Could you check a few things on this model? Use its own coordinates, in mm. Face numbers are marked on the shaded views. Give positions to 0.01 mm unless a question says otherwise; leave off trailing zeros. Order: outer loops, then holes, each group sorted by start corner. A loop starts at its lowest first (then second) coordinate and runs counter-clockwise, first axis right, second up. Notation, with made-up numbers: (37, 1.25) -> (48, 1.25) arc R15 ccw to (48, 13.25) -> close; hole circle Ø6 at (-34.75, -1). An arc over 180 degrees is marked (long way). Use one line per item in the form item = value. Start each with the question number.
from build123d import *

# Parameters (mm, degrees)
BOSS_EXTRUDE1_DEPTH     = 3.175
SKETCH2_W               = 6.35
SKETCH2_H               = 25.4
BOSS_EXTRUDE2_DEPTH     = 50.8
SKETCH3_R               = 5.207
CUT_EXTRUDE1_DEPTH      = 34.655
CUT_EXTRUDE1_DEPTH_BACK = 297.545
SKETCH4_W               = 50.8
SKETCH4_H               = 19.05
CUT_EXTRUDE2_DEPTH      = 54.975


with BuildPart() as part:
    # Sketch1 → Boss-Extrude1 (new body, symmetric)
    with BuildSketch(Plane(origin=(0, 0, 0), x_dir=(1, 0, 0), z_dir=(0, 1, 0))):
        Polygon((-136.779, 63.5), (-111.379, 63.5), (-12.7, 63.5), (-12.7, 31.75), (12.7, 31.75), (12.7, 63.5), (111.125, 63.5), (111.125, 31.75), (136.525, 31.75), (136.525, 63.5), (161.925, 63.5), (161.925, 34.874677354), (165.1, 34.874677354), (165.1, 14.046677354), (161.925, 14.046677354), (161.925, 10.414), (141.605, 10.414), (141.605, -10.414), (161.925, -10.414), (161.925, -14.046677354), (165.1, -14.046677354), (165.1, -34.874677354), (161.925, -34.874677354), (161.925, -63.5), (121.92, -63.5), (121.92, -57.15), (106.68, -57.15), (106.68, -63.5), (12.7, -63.5), (12.7, -31.75), (-12.7, -31.75), (-12.7, -63.5), (-106.68, -63.5), (-110.5408, -63.5), (-135.9408, -63.5), (-161.925, -63.5), (-161.925, -34.874677354), (-165.1, -34.874677354), (-165.1, -14.046677354), (-161.925, -14.046677354), (-161.925, -10.414), (-141.605, -10.414), (-141.605, 10.414), (-161.925, 10.414), (-161.925, 14.046677354), (-165.1, 14.046677354), (-165.1, 34.874677354), (-161.925, 34.874677354), (-161.925, 63.5), align=None)
    extrude(amount=BOSS_EXTRUDE1_DEPTH, both=True)

    # Sketch2 → Boss-Extrude2 (add, symmetric)
    with BuildSketch(Plane(origin=(0, 0, 0), x_dir=(1, 0, 0), z_dir=(0, 1, 0))):
        with Locations((128.27, 0)):
            Rectangle(SKETCH2_W, SKETCH2_H)
        with Locations((-128.27, 0)):
            Rectangle(SKETCH2_W, SKETCH2_H)
    extrude(amount=BOSS_EXTRUDE2_DEPTH, both=True)

    # Sketch3 → Cut-Extrude1 (cut, two sides)
    with BuildSketch(Plane.ZY.offset(131.445)) as cut_extrude1_sk:
        with Locations((0, 43.18)):
            Circle(SKETCH3_R)
        with Locations((0, -43.18)):
            Circle(SKETCH3_R)
    extrude(amount=CUT_EXTRUDE1_DEPTH, mode=Mode.SUBTRACT)
    extrude(cut_extrude1_sk.sketch, amount=-CUT_EXTRUDE1_DEPTH_BACK, mode=Mode.SUBTRACT)

    # Sketch4 → Cut-Extrude2 (cut, through all)
    with BuildSketch(Plane(origin=(0, 3.175, 0), x_dir=(1, 0, 0), z_dir=(0, 1, 0))):
        with Locations((-50.8, 53.975)):
            Rectangle(SKETCH4_W, SKETCH4_H)
    extrude(amount=-CUT_EXTRUDE2_DEPTH, mode=Mode.SUBTRACT)


solid = part.part
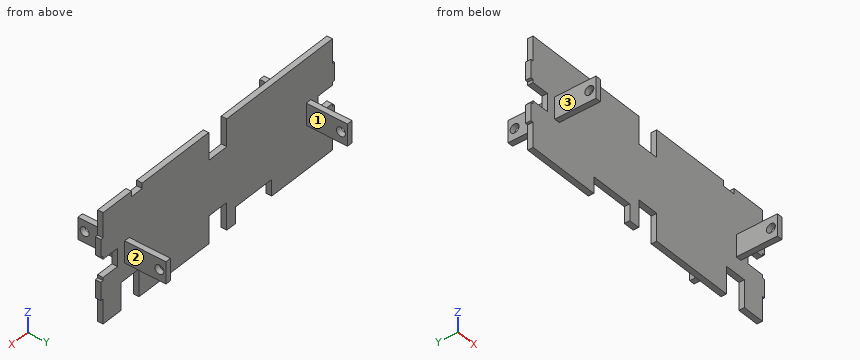
(1) Imagine slicing it at C-C (y = 24). Write out the boundary of the cut face in (x, z) (3 decimals), plus the area to 3 significant figures.
(2) I'm going to push flat-ended pins straight in: pin 1 Ø1.6 at (x, y) = (-163.5, -0.5) entering from +Z; pin 2 Ø5 at (y, z) = (-1, -51) entering from +X (3 decimals); pin 3 Ø1.6 at (x, y) = (163.5, 1) entering from -Z; pin 4 Ø12 at (x, z) = (121, -40) entering from +Y. Where does each tip first touch, or does it pass through?
(3) Imagine slicing it at D-D (x = -29). Write out the boundary of the cut face in (y, z) (3 decimals).
(4) Imagine slicing it at B-B (y = -43.18). Write out the boundary of the cut face in (x, z) (3 decimals), plus the area to 3 significant figures.
(5) Please list where these lines run through material, in increasing order: probe 1 along X at (y, z) = (2, -32.5) (3 decimals); probe 2 along Y at (x, z) = (127, 0); probe 3 along X at (y, z) = (33, 11.5) (3 decimals).
(6) We'd pull the mould along X, two halves only. Please class the marked faces 1, 2 and 3: pulls with the +X half, pulls with the -X half, needs draft (parallel to the pull), parting line crosses it, or undercut.
(7) Imagine slicing it at A-A (z = -50). Write out the boundary of the cut face in (x, y) (3 decimals), plus the area to 3 significant figures.
Calculated:
q1.outline = (-131.445, -12.7) -> (-125.095, -12.7) -> (-125.095, 12.7) -> (-131.445, 12.7) -> close; (125.095, -12.7) -> (131.445, -12.7) -> (131.445, 12.7) -> (125.095, 12.7) -> close
q1.area = 323 mm2
q2.pin_1 = 34.87
q2.pin_2 = 161.925
q2.pin_3 = -34.87
q2.pin_4 = through
q3.outline = (-3.175, -44.45) -> (3.175, -44.45) -> (3.175, 63.5) -> (-3.175, 63.5) -> close
q4.outline = (-131.445, -12.7) -> (-125.095, -12.7) -> (-125.095, -5.207) -> (-131.445, -5.207) -> close; (-131.445, 5.207) -> (-125.095, 5.207) -> (-125.095, 12.7) -> (-131.445, 12.7) -> close; (125.095, -12.7) -> (131.445, -12.7) -> (131.445, -5.207) -> (125.095, -5.207) -> close; (125.095, 5.207) -> (131.445, 5.207) -> (131.445, 12.7) -> (125.095, 12.7) -> close
q4.area = 190 mm2
q5.probe_1 = -165.1 to -12.7, 12.7 to 111.125, 136.525 to 165.1
q5.probe_2 = -50.8 to -48.39, -37.97 to 37.97, 48.39 to 50.8
q5.probe_3 = -131.445 to -125.095, 125.095 to 131.445
q6.face_1 = undercut
q6.face_2 = pulls with the +X half
q6.face_3 = pulls with the -X half
q7.outline = (-161.925, -3.175) -> (-76.2, -3.175) -> (-76.2, 3.175) -> (-161.925, 3.175) -> close; (-25.4, -3.175) -> (-12.7, -3.175) -> (-12.7, 3.175) -> (-25.4, 3.175) -> close; (12.7, -3.175) -> (111.125, -3.175) -> (111.125, 3.175) -> (12.7, 3.175) -> close; (136.525, -3.175) -> (161.925, -3.175) -> (161.925, 3.175) -> (136.525, 3.175) -> close
q7.area = 1,410 mm2
